The listing builds one solid part. Answer for the finished solid, in the listing's coordinates (mm). A direction names the side the tool comes from. Give positions to 0.01 mm unless a question says otherwise; leave off trailing zeros. Order: outer loops, then holes, each group sorted by start corner. A loop starts at its lowest first (then second) coordinate and runs counter-clockwise, first axis right, second up. Notation, with made-up numbers: (67, 60.5) - (76, 60.5) arc R21 cw to (76, 82.5) - close; hole circle Ø11 at (46, 85). An arc over 180 degrees is marked (long way). Answer as CSV lines item,"result". Start each with the question number.
1. Section A-A on z = 2.5 is taken. Give the vertices of the cut face in (x, y).
2. Consider line 1 along X through (y, z) = (1.5, 5); line 2 along Y through (x, z) = (-41.5, 2.5); line 3 along Y through (x, z) = (-45, 2.5). Determine where each line is inside the solid, lowest interval first. Write a range as [from, to].
3. Section C-C on x = -51 is taken. Give the vertices of the cut face in (y, z) (3 decimals).
4. Flat-ended cylindrical pins translate along their axes: pin 1 (1.5 mm diameter, centred on x = -50.5, z = 5.5, fed in from +Y); pin 2 (1 mm diameter, centred on x = -32.5, z = 1, fed in from +Y). Find the tip coordinate at first contact, or state that the pin passes through.
5. Section B-B on y = 1 is taken. Give the vertices of the cut face in (x, z), and give its area (3 significant figures).
6. Section D-D on z = 5.5 is taken. Give the vertices of the cut face in (x, y).
7. Determine the mould class of faces 1 (the flat face through (-58.72, 2.5, 1.8)), 2 (the cylindrical face through (-49.062, 4.434, 3.34)), 3 (the flat face through (-29, 0, 2)) for opening direction X: +X half, -X half, draft (parallel to the pull), parting line (faces both ways), or undercut.
8. Which of the six approach directions +Z, -Z, +X, -X, +Y, -Y give full straight-line access (tool end or side, diameter ignored) to faces 4 (the cylindrical face through (-29.22, 0.95, 5.44)), 5 (the flat face through (-55.334, -9.304, 3.131))?
from build123d import *

# Parameters (mm, degrees)
BOSS_EXTRUDE1_DEPTH = 6.35
SKETCH3_R           = 3.175
SKETCH3_R_2         = 1.27
BOSS_EXTRUDE3_DEPTH = 58.720417
CUT_EXTRUDE3_START  = -19.05
SKETCH3_7_R         = 3.175
SKETCH3_7_R_2       = 1.27
CUT_EXTRUDE3_DEPTH  = 20.620416805


with BuildPart() as part:
    # Sketch1 → Boss-Extrude1 (new body)
    with BuildSketch(Plane.XY):
        Polygon((-51.851432898, -18.872378179), (0, 0), (-58.720416805, 0), align=None)
    extrude(amount=BOSS_EXTRUDE1_DEPTH)

    # Sketch3 → Boss-Extrude3 (add)
    with BuildSketch(Plane(origin=(0, 0, 0), x_dir=(0, 0, -1), z_dir=(1, 0, 0))):
        with Locations((-3.175, 3.175)):
            Circle(SKETCH3_R)
        with Locations((-3.175, 3.175)):
            Circle(SKETCH3_R_2, mode=Mode.SUBTRACT)
        with BuildLine():
            Line((0, 0), (0, 3.175))
            ThreePointArc((0, 3.175), (-0.92993597, 0.92993597), (-3.175, 0))
            Line((-3.175, 0), (0, 0))
        make_face()
        with BuildLine():
            Line((0, 6.35), (-3.175, 6.35))
            ThreePointArc((-3.175, 6.35), (-0.92993597, 5.42006403), (0, 3.175))
            Line((0, 3.175), (0, 6.35))
        make_face()
        with BuildLine():
            ThreePointArc((-3.175, 0), (-5.42006403, 0.92993597), (-6.35, 3.175))
            Line((-6.35, 3.175), (-6.35, 0))
            Line((-6.35, 0), (-3.175, 0))
        make_face()
    extrude(amount=-BOSS_EXTRUDE3_DEPTH)

    # Sketch3<7> → Cut-Extrude3 (cut)
    with BuildSketch(Plane(origin=(0, 0, 0), x_dir=(0, 0, -1), z_dir=(1, 0, 0)).offset(CUT_EXTRUDE3_START)):
        with Locations((-3.175, 3.175)):
            Circle(SKETCH3_7_R)
        with Locations((-3.175, 3.175)):
            Circle(SKETCH3_7_R_2, mode=Mode.SUBTRACT)
        with BuildLine():
            Line((0, 6.35), (-3.175, 6.35))
            ThreePointArc((-3.175, 6.35), (-0.92993597, 5.42006403), (0, 3.175))
            Line((0, 3.175), (0, 6.35))
        make_face()
        with BuildLine():
            Line((0, 0), (0, 3.175))
            ThreePointArc((0, 3.175), (-0.92993597, 0.92993597), (-3.175, 0))
            Line((-3.175, 0), (0, 0))
        make_face()
    extrude(amount=-CUT_EXTRUDE3_DEPTH, mode=Mode.SUBTRACT)


solid = part.part
Checks:
1,outline,"(-58.72, 0) - (-51.85, -18.87) - (0, 0) - (0, 2.1) - (-19.05, 2.1) - (-19.05, 0) - (-39.67, 0) - (-39.67, 2.1) - (-58.72, 2.1) - close; (-58.72, 4.25) - (-39.67, 4.25) - (-39.67, 6.35) - (-58.72, 6.35) - close; (-19.05, 4.25) - (0, 4.25) - (0, 6.35) - (-19.05, 6.35) - close"
2,line 1,"x = [-58.72, -39.67], [-19.05, 0]"
2,line 2,"y = [-15.1, 2.1], [4.25, 6.35]"
2,line 3,"y = [-16.38, 2.1], [4.25, 6.35]"
3,outline,"(-18.562, 0) - (6.35, 0) - (6.35, 3.175) arc R3.175 ccw to (3.175, 6.35) - (-18.562, 6.35) - close; hole circle Ø2.54 at (3.175, 3.175)"
4,pin 1,"stops at y = 5.93"
4,pin 2,"stops at y = 0"
5,outline,"(-58.72, 0) - (-39.67, 0) - (-39.67, 5.49) - (-19.05, 5.49) - (-19.05, 0) - (0, 0) - (0, 6.35) - (-58.72, 6.35) - close"
5,area,"260 mm²"
6,outline,"(-58.72, 0) - (-51.85, -18.87) - (0, 0) - (0, 5.34) - (-19.05, 5.34) - (-19.05, 1.01) - (-39.67, 1.01) - (-39.67, 5.34) - (-58.72, 5.34) - close"
7,face 1,"-X half"
7,face 2,"draft"
7,face 3,"undercut"
8,face 4,"-Z, +Y"
8,face 5,"+Z, -Z, -X, -Y"
